Part model, mm, in its own coordinate system. A direction names the side the tool comes from. Coordinates: 2 decimals unless noted, no trailing zeros. Loops run counter-clockwise (first coordinate to the right, second up) from the corner with the lowest first, then second, coordinate; pieces in that order, holes last. Notation, with made-up numbers: (12.5, 32) - (71.5, 32) arc R11 ccw to (71.5, 37) - close; hole circle Ø11 at (30, 48). An arc over 180 degrees is marked (long way). Answer as CSV lines item,"result".
Autodesk Inventor part; units mm, degrees
ref_plane "YZ Plane" through (0, 0, 0) normal (1, 0, 0) x (0, 1, 0)
ref_plane "XZ Plane" through (0, 0, 0) normal (0, 1, 0) x (-1, 0, 0)
ref_plane "XY Plane" through (0, 0, 0) normal (0, 0, 1) x (1, 0, 0)
sketch "Szkic1" plane through (0, 0, 0) normal (0, 0, 1) x (1, 0, 0)
  line L0 (-18.8999, 4.9578) -> (17.1001, 4.9578)
  line L1 (17.1001, 4.9578) -> (17.1001, -45.0422)
  line L2 (17.1001, -45.0422) -> (-18.8999, -45.0422)
  line L3 (-18.8999, -45.0422) -> (-18.8999, 4.9578)
  point P0 (0, 0)
  dimension "d0" = 36
  dimension "d1" = 50
extrude "Wyciągnięcie proste1" add sketch "Szkic1" along normal blind 40
sketch "Szkic2" plane through (0, 0, 40) normal (0, 0, 1) x (1, 0, 0)
  line L0 (-18.8999, 4.9578) -> (-18.8999, -45.0422)
  line L1 (-18.8999, -45.0422) -> (17.1001, -45.0422)
  line L2 (-18.8999, 4.9578) -> (17.1001, -45.0422)
  line L3 (17.1001, -45.0422) -> (17.1001, 4.9578)
  line L4 (17.1001, 4.9578) -> (-18.8999, -45.0422)
  circle A0 centre (-0.8999, -20.0422) radius 10
  point P0 (0, 0)
  dimension "d4" = 20
extrude "Wyciągnięcie proste2" add sketch "Szkic2" along normal blind 70 contours A0 L4 L2 | L2 L4 A0 | L4 L2 A0 | L4 A0 L2
mirror "Odbij1" about plane through (-0.8999, -20.0422, 0) normal (0, 0, -1)
sketch "Szkic3" plane through (17.1001, -45.0422, 40) normal (1, 0, 0) x (0, 0, -1)
  line L0 (0, 0) -> (0, 50)
  line L1 (80, 0) -> (0, 0)
  line L2 (0, 50) -> (80, 0)
  line L3 (80, 0) -> (80, 50)
  line L4 (80, 50) -> (0, 0)
  point P0 (40, 45.0422)
  point P1 (40, 25)
hole "Otwór1" at (17.1001, -20.0422, 0) direction (-1, 0, 0) diameter 27 end through all
properties part number "sworzeń z nakrętką"
Q1. Two-plate mould, pull along Y, no slides. Class faces 1 (the face through (7.4, -14.1, -40)), 2 (the face through (-1.152, -6.863, 2.927)), 3 (the face through (-8.836, -26.127, -74.51)), 4 (the face through (-1, -45.042, -1)): released by +Y, released by -Y, zero draft, split by the parting line, or undercut.
Results:
face 1,"zero draft"
face 2,"undercut"
face 3,"split by the parting line"
face 4,"released by -Y"
Q2. Wall check: L1, parallel to Y at x = -7, z = 0; L2, parallel to Z at x = -14.5, y = -32; L3, parallel to Z at x = 3, y = -27.5. Give the ranges that are in metal, low to high.
Results:
L1,"y = -45.04 to -33.54, -6.54 to 4.96"
L2,"z = -40 to -6.27, 6.27 to 40"
L3,"z = -110 to -11.25, 11.25 to 110"
Q3. Flat gauge pins, fed straight in: pin 1 (5 mm diameter, centred on x = 10.5, z = -44.5, fed in from -Y); pin 2 (10 mm diameter, centred on x = -4, z = 65.5, fed in from -Y); pin 3 (8 mm diameter, centred on x = 2, y = -39, fed in from -Z). Where does each tip first touch, or does it go through?
Results:
pin 1,"stops at y = -24.6"
pin 2,"stops at y = -30.04"
pin 3,"stops at z = -40"
Q4. Saw through at C-C (x = -8). Give the cut face in (y, z).
Results:
outline,"(-45.04, -40) - (-27.08, -40) - (-27.08, -110) - (-13, -110) - (-13, -40) - (4.96, -40) - (4.96, 40) - (-13, 40) - (-13, 110) - (-27.08, 110) - (-27.08, 40) - (-45.04, 40) - close; hole circle Ø27 at (-20.04, 0)"
Q5. Saw through at D-D (y = -41). Give the cut face in (x, z).
Results:
outline,"(-18.9, -40) - (17.1, -40) - (17.1, 40) - (-18.9, 40) - close"
Q6. Saw through at A-A (z = 0). Give the cut face in (x, y).
Results:
outline,"(-18.9, -45.04) - (17.1, -45.04) - (17.1, -33.54) - (-18.9, -33.54) - close; (-18.9, -6.54) - (17.1, -6.54) - (17.1, 4.96) - (-18.9, 4.96) - close"
Q7. Which spindle directions (+Z, -Z, +X, -X, +Y, -Y) get a long thin tool onto all of the face, cutting with end or side? Do faces 5 (the face through (-1, -20, -110)), 6 (the face through (-2.202, -29.957, 74.51)). Say none if no direction does.
Results:
face 5,"-Z, +X, -X, +Y, -Y"
face 6,"+Z"
Q8. Saw through at B-B (y = -17.5). Give the cut face in (x, z).
Results:
outline,"(-18.9, -40) - (-10.57, -40) - (-10.57, -110) - (8.77, -110) - (8.77, -40) - (17.1, -40) - (17.1, -13.26) - (-18.9, -13.26) - close; (-18.9, 13.26) - (17.1, 13.26) - (17.1, 40) - (8.77, 40) - (8.77, 110) - (-10.57, 110) - (-10.57, 40) - (-18.9, 40) - close"
